```python
from build123d import *

# Parameters (mm, degrees)
SKETCH1_W           = 100
SKETCH1_H           = 30
BOSS_EXTRUDE1_DEPTH = 60
SKETCH2_R           = 25
BOSS_EXTRUDE2_DEPTH = 20
SKETCH3_R           = 10
SKETCH3_W           = 10
SKETCH3_H           = 10
BOSS_EXTRUDE3_DEPTH = 5
SKETCH4_W           = 30
SKETCH4_H           = 30
BOSS_EXTRUDE4_DEPTH = 10
CHAMFER1_SIZE       = 10
FILLET1_R           = 1
FILLET2_R           = 1.5
FILLET3_R           = 3.5
SKETCH5_R           = 10.925128043
CUT_EXTRUDE1_DEPTH  = 5
CUT_EXTRUDE1_TAPER  = 28


with BuildPart() as part:
    # Sketch1 → Boss-Extrude1 (new body)
    with BuildSketch(Plane(origin=(0, 0, 0), x_dir=(1, 0, 0), z_dir=(0, 1, 0))):
        with Locations((50, 15)):
            Rectangle(SKETCH1_W, SKETCH1_H)
    extrude(amount=BOSS_EXTRUDE1_DEPTH)

    # Sketch2 → Boss-Extrude2 (add)
    with BuildSketch(Plane.XY):
        with Locations((50, 30)):
            Circle(SKETCH2_R)
    extrude(amount=BOSS_EXTRUDE2_DEPTH)

    # Sketch3 → Boss-Extrude3 (add)
    with BuildSketch(Plane(origin=(0, 60, 0), x_dir=(1, 0, 0), z_dir=(0, 1, 0))):
        with Locations((85, 15)):
            Circle(SKETCH3_R)
        with Locations((15, 15)):
            Rectangle(SKETCH3_W, SKETCH3_H)
    extrude(amount=BOSS_EXTRUDE3_DEPTH)

    # Sketch4 → Boss-Extrude4 (add)
    with BuildSketch(Plane(origin=(0, 60, 0), x_dir=(1, 0, 0), z_dir=(0, 1, 0))):
        with Locations((50, 15)):
            Rectangle(SKETCH4_W, SKETCH4_H)
    extrude(amount=BOSS_EXTRUDE4_DEPTH)

    # Chamfer1
    chamfer1_edges = [part.edges().sort_by_distance(p)[0] for p in [
        (50, 70, 0),
    ]]
    chamfer(chamfer1_edges, length=CHAMFER1_SIZE)

    # Fillet1
    fillet1_edges = [part.edges().sort_by_distance(p)[0] for p in [
        (20, 62.5, -10),
        (20, 62.5, -20),
        (10, 62.5, -20),
        (10, 62.5, -10),
        (20, 65, -15),
        (15, 65, -20),
        (10, 65, -15),
        (15, 65, -10),
    ]]
    fillet(fillet1_edges, radius=FILLET1_R)

    # Fillet2
    fillet2_edges = [part.edges().sort_by_distance(p)[0] for p in [
        (75, 65, -15),
    ]]
    fillet(fillet2_edges, radius=FILLET2_R)

    # Fillet3
    fillet3_edges = [part.edges().sort_by_distance(p)[0] for p in [
        (25, 30, 0),
        (25, 30, 20),
    ]]
    fillet(fillet3_edges, radius=FILLET3_R)

    # Sketch5 → Cut-Extrude1 (cut)
    with BuildSketch(Plane.XY.offset(20)):
        with Locations((50, 30)):
            Circle(SKETCH5_R)
    extrude(amount=-CUT_EXTRUDE1_DEPTH, taper=CUT_EXTRUDE1_TAPER, mode=Mode.SUBTRACT)


solid = part.part
```
Can you work these out from the model? Positions are in its coordinate system, mm. A direction names the side the tool comes from. Coordinates: 2 decimals unless noted, no trailing zeros. Write each loop counter-clockwise with the first axis right and the second up, starting at its lowest first coordinate (ties: lowest second). Pieces come first, ordered by that corner, then holes. Notation, with made-up numbers: (68, 59) - (109, 59) arc R10 cw to (109, 76) - close; hole circle Ø3 at (64, 6). An arc over 180 degrees is marked (long way). Return JSON: item names as keys, results as strings.
Q1. If we section it at A-A (x = 50): Please give me the cut outline in (y, z), then the cut area to 3 significant figures.
Computed values:
{"outline": "(0, -30) - (70, -30) - (70, -10) - (60, 0) - (58.5, 0) arc R3.5 cw to (55, 3.5) - (55, 16.5) arc R3.5 ccw to (51.5, 20) - (40.93, 20) - (38.27, 15) - (21.73, 15) - (19.07, 20) - (8.5, 20) arc R3.5 ccw to (5, 16.5) - (5, 3.5) arc R3.5 cw to (1.5, 0) - (0, 0) - close", "area": "2,950 mm2"}
Q2. Please list where these lines run through material, in increasing order: L1, parallel to X at y = 62, z = -18.5; L2, parallel to Z at x = 83, y = 30; L3, parallel to Y at x = 78, z = -13. Write a range as from..to.
Computed values:
{"L1": "x = 10..20, 35..65, 75.63..94.37", "L2": "z = -30..0", "L3": "y = 0..65"}
Q3. If we section it at C-C (x = 85): Please give me the cut outline in (y, z), then the cut area to 3 significant figures.
Computed values:
{"outline": "(0, -30) - (60, -30) - (60, -25) - (63.5, -25) arc R1.5 ccw to (65, -23.5) - (65, -6.5) arc R1.5 ccw to (63.5, -5) - (60, -5) - (60, 0) - (0, 0) - close", "area": "1,900 mm2"}
Q4. If we section it at B-B (z = -15): Please give me the cut outline in (x, y).
Computed values:
{"outline": "(0, 0) - (100, 0) - (100, 60) - (95, 60) - (95, 63.5) arc R1.5 ccw to (93.5, 65) - (76.5, 65) arc R1.5 ccw to (75, 63.5) - (75, 60) - (65, 60) - (65, 70) - (35, 70) - (35, 60) - (20, 60) - (20, 64) arc R1 ccw to (19, 65) - (11, 65) arc R1 ccw to (10, 64) - (10, 60) - (0, 60) - close"}
Q5. On a 3-axis mill with a long thin cutter (end or side, diameter ignored), from which of +Z, -Z, +X, -X, +Y, -Y can I reach the whole of each face in a straight line? I mean faces 4 (the flat face through (50, 30, 15)), 5 (the flat face through (85, 65, -15)), 6 (the flat face through (65, 65, -18)). Say none if no direction works.
Computed values:
{"face 4": "+Z", "face 5": "+Z, -Z, +X, +Y", "face 6": "+Z, -Z, +Y"}
Q6. If we section it at D-D (x = 15): Please give me the cut outline in (y, z).
Computed values:
{"outline": "(0, -30) - (60, -30) - (60, -20) - (64, -20) arc R1 ccw to (65, -19) - (65, -11) arc R1 ccw to (64, -10) - (60, -10) - (60, 0) - (0, 0) - close"}
Q7. Thinking about a two-plate mould opening in X: for faces 1 (the flat face through (20, 62, -15)), 2 (the flat face through (15, 62, -20)), 3 (the cylindrical face through (30, 15, 10)), which applies, +X half, -X half, draft (parallel to the pull), parting line (faces both ways), or undercut?
Computed values:
{"face 1": "undercut", "face 2": "draft", "face 3": "parting line"}
Q8. I'm going to push flat-ended pins straight in: pin 1 Ø8.5 at (x, z) = (83, -13) entering from +Y; pin 2 Ø1.2 at (y, z) = (62.5, -14) entering from +X; pin 3 Ø12 at (x, z) = (31.5, 9.5) entering from +Y. Where does each tip first touch, or does it pass through?
Computed values:
{"pin 1": "stops at y = 65", "pin 2": "stops at x = 94.99", "pin 3": "stops at y = 51.65"}
